Source: three-view drawing plus pictorial views. Frame: mm from the lowest corner of the part. Coordinates: 2 decimals unless noted, no trailing zeros. Loops run counter-clockwise (first coordinate to the right, second up) from the corner with the lowest first, then second, coordinate; pieces in that order, holes last. Notation, with made-up numbers: M 0,5 L 17,5 A10 ccw 17,24 Z; hole C 62,81 d4. An arc over 180 degrees is marked long. Use a Markdown table: item, result. Add a question column.
1. Section B-B on x = 50.8. Output: boundary loops of the cut face in (y, z) (3 decimals), then the cut area to 3 significant figures.
2. Line query: L1, parallel to Z at x = 50.8, y = 11 (3 decimals); L2, parallel to Z at x = 50, y = 33; L3, parallel to X at y = 13, z = 10. Output: solid intervals per line, ascending. Write a range as [from, to].
3. Section C-C on z = 74. Output: boundary loops of the cut face in (x, y).
4. Section A-A on z = 50.8. Output: boundary loops of the cut face in (x, y) (3 decimals).
5. Section D-D on x = 22. Output: boundary loops of the cut face in (y, z).
6. Pin query (flat end, axial travel): pin 1 (4 mm diameter, centred on y = 24, z = 73.5, fed in from -X); pin 2 (10 mm diameter, centred on x = 53, y = 45.5, fed in from -Z); pin 3 (4 mm diameter, centred on x = 88.5, y = 14.5, fed in from +Z). Return the tip coordinate at first contact, or that it passes through.
7. Draft query along Z for the marked faces 1, 2 and 3. Return one class per face: +Z half, -Z half, draft (parallel to the pull), parting line (faces both ways), or undercut.
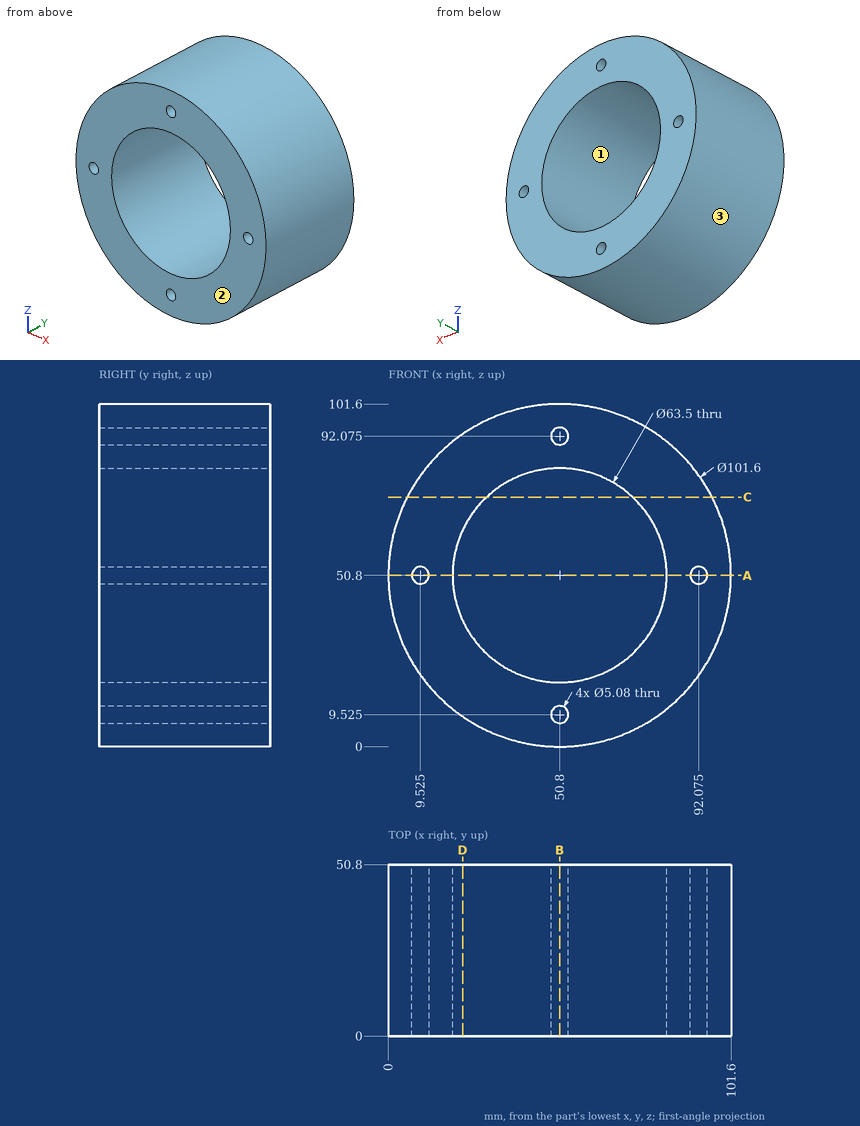
Answers below:
| question | item | result |
|---|---|---|
| 1 | outline | M 0,0 L 50.8,0 L 50.8,6.985 L 0,6.985 Z; M 0,12.065 L 50.8,12.065 L 50.8,19.05 L 0,19.05 Z; M 0,82.55 L 50.8,82.55 L 50.8,89.535 L 0,89.535 Z; M 0,94.615 L 50.8,94.615 L 50.8,101.6 L 0,101.6 Z |
| 1 | area | 1,420 mm² |
| 2 | L1 | z = [0, 6.985], [12.065, 19.05], [82.55, 89.535], [94.615, 101.6] |
| 2 | L2 | z = [0.01, 7.11], [11.94, 19.06], [82.54, 89.66], [94.49, 101.59] |
| 2 | L3 | x = [20.53, 48.3], [53.3, 81.07] |
| 3 | outline | M 5.61,0 L 29.12,0 L 29.12,50.8 L 5.61,50.8 Z; M 72.48,0 L 95.99,0 L 95.99,50.8 L 72.48,50.8 Z |
| 4 | outline | M 0,0 L 6.985,0 L 6.985,50.8 L 0,50.8 Z; M 12.065,0 L 19.05,0 L 19.05,50.8 L 12.065,50.8 Z; M 82.55,0 L 89.535,0 L 89.535,50.8 L 82.55,50.8 Z; M 94.615,0 L 101.6,0 L 101.6,50.8 L 94.615,50.8 Z |
| 5 | outline | M 0,8.95 L 50.8,8.95 L 50.8,37.44 L 0,37.44 Z; M 0,64.16 L 50.8,64.16 L 50.8,92.65 L 0,92.65 Z |
| 6 | pin 1 | stops at x = 4.41 |
| 6 | pin 2 | stops at z = 0 |
| 6 | pin 3 | stops at z = 86.94 |
| 7 | face 1 | undercut |
| 7 | face 2 | draft |
| 7 | face 3 | parting line |
